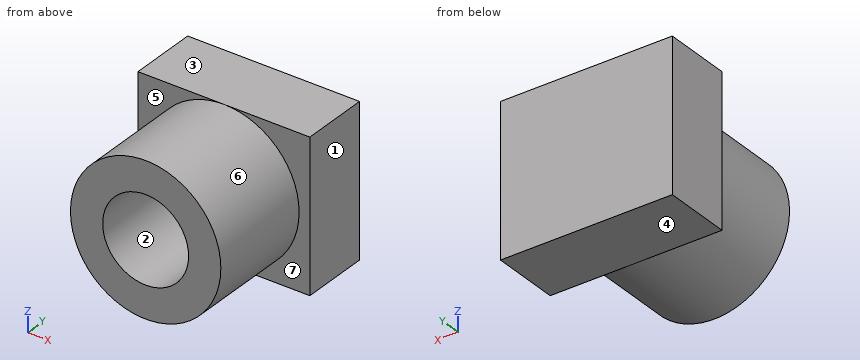
from build123d import *

# Parameters (mm, degrees)
SKETCH1_R           = 3.5
SKETCH1_R_2         = 2
BOSS_EXTRUDE1_DEPTH = 5
SKETCH2_W           = 8
SKETCH2_H           = 7
BOSS_EXTRUDE2_DEPTH = 3.175


with BuildPart() as part:
    # Sketch1 → Boss-Extrude1 (new body)
    with BuildSketch(Plane(origin=(0, 0, 0), x_dir=(1, 0, 0), z_dir=(0, 1, 0))):
        Circle(SKETCH1_R)
        Circle(SKETCH1_R_2, mode=Mode.SUBTRACT)
    extrude(amount=BOSS_EXTRUDE1_DEPTH)

    # Sketch2 → Boss-Extrude2 (add)
    with BuildSketch(Plane(origin=(0, 5, 0), x_dir=(1, 0, 0), z_dir=(0, 1, 0))):
        Rectangle(SKETCH2_W, SKETCH2_H)
    extrude(amount=BOSS_EXTRUDE2_DEPTH)


solid = part.part
Part model, mm, in its own coordinate system. Face numbers are marked on the shaded views. A direction names the side the tool comes from. Coordinates: 2 decimals unless noted, no trailing zeros. Order: outer loops, then holes, each group sorted by start corner. A loop starts at its lowest first (then second) coordinate and runs counter-clockwise, first axis right, second up. Notation, with made-up numbers: M 24.5,16.5 L 35.5,16.5 A27 ccw 35.5,36.5 Z; hole C 64.5,13.25 d11. An arc over 180 degrees is marked long. Use a Markdown table: item, result.
(1) Cut at D-D on x = -2.5. Write the cut outline in (y, z) (3 decimals).
A:
| item | result |
|---|---|
| outline | M 0,-2.449 L 5,-2.449 L 5,-3.5 L 8.175,-3.5 L 8.175,3.5 L 5,3.5 L 5,2.449 L 0,2.449 Z |
(2) Flat gauge pin, fed straight in: pin 1 (2 mm diameter, centred on y = 2, z = -0.5, fed in from -X). Where does the tip first touch, or does it go through?
A:
| item | result |
|---|---|
| pin 1 | stops at x = -3.5 |
(3) Probe L1, parallel to X at y = 3.35, z = 0; L2, parallel to Z at x = -1.5, y = 1.5. List the from-to ranges inside material, lowest first.
A:
| item | result |
|---|---|
| L1 | x = -3.5 to -2, 2 to 3.5 |
| L2 | z = -3.16 to -1.32, 1.32 to 3.16 |
(4) Pull direction Z, two halves, no side cores. Call the marked faces 1, 2 and 3: released by +Z, released by -Z, zero draft, split by the parting line, or undercut.
A:
| item | result |
|---|---|
| face 1 | zero draft |
| face 2 | undercut |
| face 3 | released by +Z |
(5) Tool access for the marked faces 4, 5, 6 and 7: list every direction of +Z, -Z, +X, -X, +Y, -Y with a clear straight run to the whole face (end or side of a thin tool).
A:
| item | result |
|---|---|
| face 4 | -Z, +X, -X, +Y, -Y |
| face 5 | -X, -Y |
| face 6 | -Y |
| face 7 | +X, -Y |
(6) Cut at C-C on y = 0.75. Write the cut outline in (x, z).
A:
| item | result |
|---|---|
| outline | C 0,0 d7; hole C 0,0 d4 |
(7) Cut at A-A on z = 0. Write the cut outline in (x, y) (3 decimals).
A:
| item | result |
|---|---|
| outline | M -4,5 L -3.5,5 L -3.5,0 L -2,0 L -2,5 L 2,5 L 2,0 L 3.5,0 L 3.5,5 L 4,5 L 4,8.175 L -4,8.175 Z |
